Geometry: final body of the model. Coordinates: model frame, mm. A direction names the side the tool comes from. Give positions to 0.01 mm unless a question says otherwise; leave off trailing zeros. Loops run counter-clockwise (first coordinate to the right, second up) from the corner with the lowest first, then second, coordinate; pieces in that order, holes last.
```python
from build123d import *

# Parameters (mm, degrees)
SKETCH1_W           = 22
SKETCH1_H           = 82.75
SKETCH1_R           = 3.1
BOSS_EXTRUDE1_DEPTH = 30
SKETCH2_W           = 22
SKETCH2_H           = 82.75
BOSS_EXTRUDE2_DEPTH = 5
SKETCH3_W           = 22
SKETCH3_H           = 14
SKETCH3_R           = 3.1
SKETCH3_W_2         = 14
SKETCH3_H_2         = 35
BOSS_EXTRUDE3_DEPTH = 5
BOSS_EXTRUDE5_START = 15
SKETCH5_R           = 3.1
BOSS_EXTRUDE5_DEPTH = 15


with BuildPart() as part:
    # Sketch1 → Boss-Extrude1 (new body)
    with BuildSketch(Plane.XY):
        with Locations((0, 7.844654309)):
            Rectangle(SKETCH1_W, SKETCH1_H)
        with Locations((0, 35.719654309)):
            Circle(SKETCH1_R, mode=Mode.SUBTRACT)
        with Locations((0, 7.719654309)):
            Circle(SKETCH1_R, mode=Mode.SUBTRACT)
    extrude(amount=BOSS_EXTRUDE1_DEPTH)

    # Sketch2 → Boss-Extrude2 (add)
    with BuildSketch(Plane.XY.offset(30)):
        with Locations((0, 7.844654309)):
            Rectangle(SKETCH2_W, SKETCH2_H)
    extrude(amount=BOSS_EXTRUDE2_DEPTH)

    # Sketch3 → Boss-Extrude3 (add)
    # profile 1 of 2: a face of its own
    with BuildSketch(Plane.XZ.offset(33.530345691)):
        with Locations((0, -7)):
            Rectangle(SKETCH3_W, SKETCH3_H)
        with Locations(Location((0, -7, 0), (0, 0, 270))):
            Circle(SKETCH3_R, mode=Mode.SUBTRACT)
    # profile 2 of 2: a face of its own
    with BuildSketch(Plane.XZ.offset(33.530345691)):
        with Locations((18, 17.5)):
            Rectangle(SKETCH3_W_2, SKETCH3_H_2)
        with Locations(Location((18, 27, 0), (0, 0, 270))):
            Circle(SKETCH3_R, mode=Mode.SUBTRACT)
        with Locations(Location((18, 8, 0), (0, 0, 270))):
            Circle(SKETCH3_R, mode=Mode.SUBTRACT)
    extrude(amount=-BOSS_EXTRUDE3_DEPTH)

    # Sketch5 → Boss-Extrude5 (add)
    with BuildSketch(Plane(origin=(0, 0, 30), x_dir=(-1, 0, 0), z_dir=(0, 0, -1)).offset(BOSS_EXTRUDE5_START)):
        with Locations((0, 7.719654309)):
            Circle(SKETCH5_R)
        with Locations((0, 35.719654309)):
            Circle(SKETCH5_R)
    extrude(amount=-BOSS_EXTRUDE5_DEPTH)


solid = part.part
```
Q1. Section query D-D, the plane y = 37. Return loops of the section in (x, z), and give its area (3 significant figures).
Q2. Mould query, pull axis Y, two halves, no side actions, for faces 5 (the face through (18.1, -31.1, 30.1)), 6 (the face through (3, -33.53, 11)), 7 (the face through (0, 49.22, 17)), 8 (the face through (0, 8, 15)). Classes: +Y half, -Y half, draft (parallel to the pull), parting line (faces both ways), or undercut.
Q3. Material intervals for probe 1 along Y at (x, z) = (0, 6); probe 2 along X at (y, z) = (-30, 8); probe 3 along Y at (x, z) = (-1, 8), sorted ascending.
Q4. Section query A-A, the plane z = 8. Return loops of the section in (x, y), and give its area (3 significant figures).
Q5. Pin query (flat end, axial travel): pin 1 Ø3 at (x, y) = (-1, 8) entering from -Z; pin 2 Ø12 at (y, z) = (41, -2) entering from +X; pin 3 Ø1 at (x, y) = (-3, -9.5) entering from -Z; pin 4 Ø5 at (x, z) = (18, 8) entering from +Y. Return the tip coordinate at first contact, or that it passes through.
Q6. Section query C-C, the plane x = 16.5. Return loops of the section in (y, z), and give its area (3 significant figures).
Q7. Section query B-B, the plane z = -7. Return loops of the section in (x, y), and give its area (3 significant figures).
Q8. Reachability of faces 1 (the face through (18, -31, 0)), 2 (the face through (-0.7, 4.7, 7.4)), 3 (the face through (0, 11, 0)), 4 (the face through (11, 10, 17)) from +Z, -Z, +X, -X, +Y, -Y: full face, straight path, thin tool, end or side. Return the list, or none.
Resolved:
1. outline: (-11, 0) - (-2.82, 0) - (-2.82, 15) - (2.82, 15) - (2.82, 0) - (11, 0) - (11, 35) - (-11, 35) - close
1. area: 685 mm2
2. face 5: draft
2. face 6: -Y half
2. face 7: +Y half
2. face 8: undercut
3. probe 1: y = -33.53 to 4.62, 10.82 to 32.62, 38.82 to 49.22
3. probe 2: x = -11 to 14.9, 21.1 to 25
3. probe 3: y = -33.53 to 4.79, 10.65 to 32.79, 38.65 to 49.22
4. outline: (-11, -33.53) - (14.9, -33.53) - (14.9, -28.53) - (11, -28.53) - (11, 49.22) - (-11, 49.22) - close; (21.1, -33.53) - (25, -33.53) - (25, -28.53) - (21.1, -28.53) - close; hole circle Ø6.2 at (0, 7.72); hole circle Ø6.2 at (0, 35.72)
4. area: 1,800 mm2
5. pin 1: stops at z = 15
5. pin 2: stops at x = 11
5. pin 3: stops at z = 0
5. pin 4: passes through
6. outline: (-33.53, 0) - (-28.53, 0) - (-28.53, 5.29) - (-33.53, 5.29) - close; (-33.53, 10.71) - (-28.53, 10.71) - (-28.53, 24.29) - (-33.53, 24.29) - close; (-33.53, 29.71) - (-28.53, 29.71) - (-28.53, 35) - (-33.53, 35) - close
6. area: 121 mm2
7. outline: (-11, -33.53) - (-3.1, -33.53) - (-3.1, -28.53) - (-11, -28.53) - close; (3.1, -33.53) - (11, -33.53) - (11, -28.53) - (3.1, -28.53) - close
7. area: 79.0 mm2
8. face 1: -Z, +X, +Y, -Y
8. face 2: -Z
8. face 3: -Z, +X, -X, +Y
8. face 4: +Z, -Z, +X, +Y
